Input: dimensioned drawing with shaded views. Units: mm. Origin: part minimum x, y, z. A direction names the side the tool comes from. Give positions to 0.01 mm unless a question says otherwise; leave off trailing zeros. Write each loop counter-clockwise with the first axis right and the second up, starting at its lowest first coordinate (ties: lowest second). Pieces come first, ordered by that corner, then holes. Notation, with made-up numbers: (-2, 42) - (16, 42) arc R27 cw to (16, 66) - close; hole circle Ø11 at (-26.75, -22.5). An arc over 180 degrees is marked (long way). Answer as CSV lines item,"result".
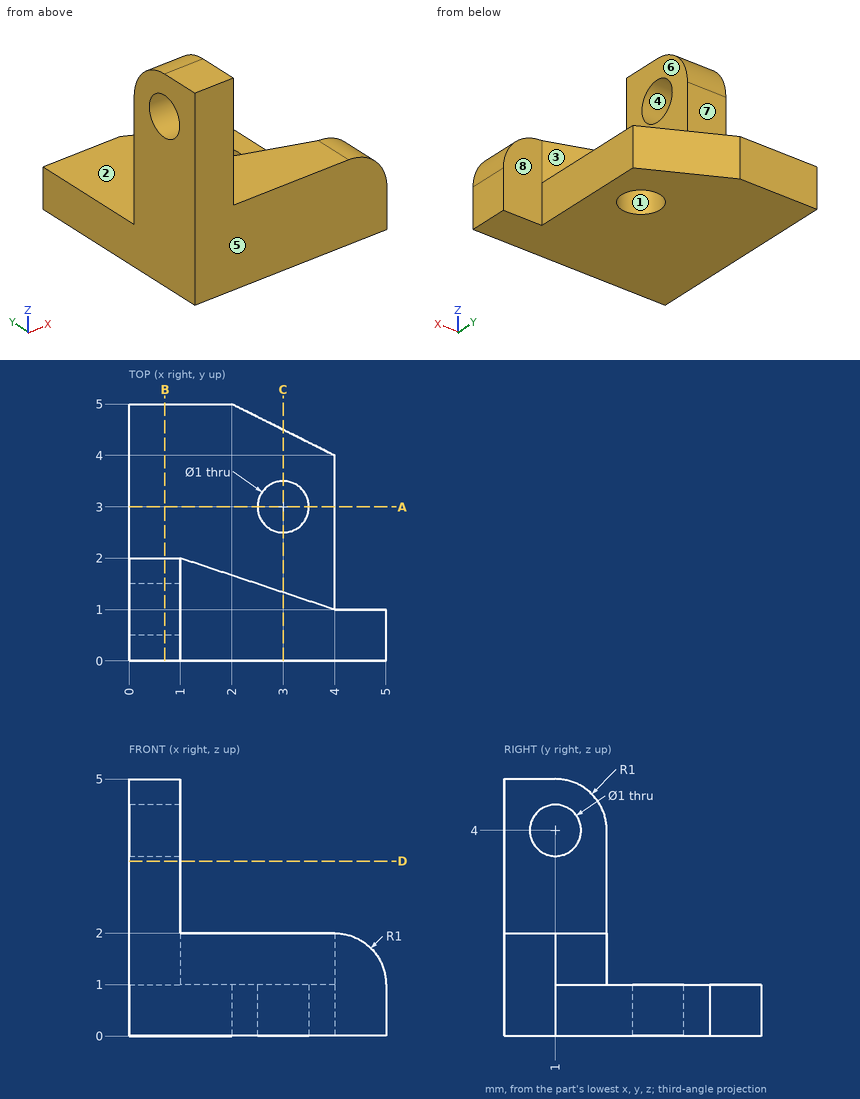
Item 1: Ray query, line 1 (Z direction, x = 3.7, y = 2.05); line 2 (Y direction, x = 0.9, z = 3.85). Return the intervals inside material, ascending. Write a range as from..to.
The answers:
line 1,"0..1"
line 2,"0..0.52, 1.48..2"
Item 2: Cut plane C-C on x = 3. Return the cut outline in (y, z), plus the area to 3 significant figures.
The answers:
outline,"(0, 0) - (2.5, 0) - (2.5, 1) - (1.33, 1) - (1.33, 2) - (0, 2) - close; (3.5, 0) - (4.5, 0) - (4.5, 1) - (3.5, 1) - close"
area,"4.83 mm²"
Item 3: Cut plane B-B on x = 0.7. Return the cut outline in (y, z).
The answers:
outline,"(0, 0) - (5, 0) - (5, 1) - (2, 1) - (2, 4) arc R1 ccw to (1, 5) - (0, 5) - close; hole circle Ø1 at (1, 4)"
Item 4: Reachability of the marked faces 5, 6, 7 and 8 from +Z, -Z, +X, -X, +Y, -Y: full face, straight path, thin tool, end or side. Return the list, or none.
The answers:
face 5,"+Z, -Z, +X, -X, -Y"
face 6,"+Z, +X, +Y, -Y"
face 7,"+Z, +X, -X, +Y"
face 8,"+Z, -Z, +X, +Y"
Item 5: Cut plane D-D on z = 3.4. Return the cut outline in (x, y), plus the area to 3 significant figures.
The answers:
outline,"(0, 0) - (1, 0) - (1, 2) - (0, 2) - close"
area,"2.00 mm²"
Item 6: Cut plane A-A on y = 3. Return the cut outline in (x, z), plus the area to 3 significant figures.
The answers:
outline,"(0, 0) - (2.5, 0) - (2.5, 1) - (0, 1) - close; (3.5, 0) - (4, 0) - (4, 1) - (3.5, 1) - close"
area,"3.00 mm²"
Item 7: Mould query, pull axis Y, two halves, no side actions, for the marked faces 1, 2, 3 and 4. Classes: +Y half, -Y half, draft (parallel to the pull), parting line (faces both ways), or undercut.
The answers:
face 1,"undercut"
face 2,"draft"
face 3,"+Y half"
face 4,"undercut"
Item 8: Contact query for flat-ended pins moving along their axis: pin 1 (1.5 mm diameter, centred on x = 0.5, z = 3, fed in from +Y); pin 2 (1 mm diameter, centred on x = 3, y = 0.5, fed in from +Z); pin 3 (1.6 mm diameter, centred on y = 0.5, z = 3.5, fed in from +X). Output: stop coordinate, or through.
The answers:
pin 1,"y = 2"
pin 2,"z = 2"
pin 3,"x = 1"
